Read the model definition and answer for the solid it produces. Units are mm, in the model's axes. Face numbers are marked on the shaded views. Coordinates: 2 decimals unless noted, no trailing zeros. Write each loop counter-clockwise with the first axis right and the second up, starting at its lowest first coordinate (ties: lowest second). Pieces come first, ordered by that corner, then holes.
(1) The part is cut by section D-D, the plane z = -8. Determine the outline of the cut face in (x, y), and give its area (3 significant figures).
(2) The part is cut by section C-C, the plane x = -14.25. Determine the outline of the cut face in (y, z), and give its area (3 significant figures).
(3) The part is cut by section A-A, the plane x = 0. Determine the outline of the cut face in (y, z).
(4) Given pin 1 (3 mm diameter, centred on y = 69, z = -3, fed in from -X); pin 2 (4 mm diameter, centred on y = 16, z = -0.5, fed in from -X), each flat-ended and moving along its own axis, determine where each tip first touches the part or whether it passes through.
(5) Straight lines are drawn through the part: line 1 along Z through (x, y) = (0.5, 81); line 2 along Y through (x, z) = (0, 0.65); line 3 along X through (y, z) = (60, -0.5). For each, find the intervals that lie inside material, in ascending order.
(6) The part is cut by section B-B, the plane y = -17.5. Determine the outline of the cut face in (x, z), and give its area (3 significant figures).
(7) Determine the mould class of the marked faces 1, 2, 3 and 4 for opening direction Z: pulls with the +Z half, pulls with the -Z half, needs draft (parallel to the pull), parting line crosses it, or undercut.
```python
from build123d import *

# Parameters (mm, degrees)
F0_W     = 30
F0_H     = 126.4803184569
F1_DEPTH = 3
F2_W     = 3
F2_H     = 126.4803184569
F3_DEPTH = 30
F4_START = -24
F4_DEPTH = 3


with BuildPart() as f1:
    # F0 (on Top) → F1 (new body)
    with BuildSketch(Plane.XY):
        with Locations((-3, 28.2401592284)):
            Rectangle(F0_W, F0_H)
        with BuildLine():
            ThreePointArc((-6.2781745931, -7.7781745931), (-9.1639938918, -8.3521997416), (-6.7175144213, -6.7175144213))
            ThreePointArc((-6.7175144213, -6.7175144213), (-6.3923552943, -7.2041494445), (-6.2781745931, -7.7781745931))
        make_face(mode=Mode.SUBTRACT)
        with BuildLine():
            ThreePointArc((-3.5355339059, -3.5355339059), (-1.9134171618, 4.6193976626), (5, 0))
            ThreePointArc((5, 0), (1.9134171618, -4.6193976626), (-3.5355339059, -3.5355339059))
        make_face(mode=Mode.SUBTRACT)
    extrude(amount=F1_DEPTH)

    # F2 (on face) → F3 (join)
    with BuildSketch(Plane.XY.offset(3)):
        with Locations((10.5, 28.2401592284)):
            Rectangle(F2_W, F2_H)
    extrude(amount=-F3_DEPTH)

    # F0 (on Top) → F4 (join)
    with BuildSketch(Plane.XY.offset(F4_START)):
        with Locations((-3, 28.2401592284)):
            Rectangle(F0_W, F0_H)
        with BuildLine():
            ThreePointArc((-6.2781745931, -7.7781745931), (-9.1639938918, -8.3521997416), (-6.7175144213, -6.7175144213))
            ThreePointArc((-6.7175144213, -6.7175144213), (-6.3923552943, -7.2041494445), (-6.2781745931, -7.7781745931))
        make_face(mode=Mode.SUBTRACT)
        with BuildLine():
            ThreePointArc((-3.5355339059, -3.5355339059), (-1.9134171618, 4.6193976626), (5, 0))
            ThreePointArc((5, 0), (1.9134171618, -4.6193976626), (-3.5355339059, -3.5355339059))
        make_face(mode=Mode.SUBTRACT)
        with BuildLine():
            ThreePointArc((-3.5355339059, -3.5355339059), (1.9134171618, -4.6193976626), (5, 0))
            ThreePointArc((5, 0), (-1.9134171618, 4.6193976626), (-3.5355339059, -3.5355339059))
        make_face()
        with BuildLine():
            ThreePointArc((-6.2781745931, -7.7781745931), (-6.3923552943, -7.2041494445), (-6.7175144213, -6.7175144213))
            ThreePointArc((-6.7175144213, -6.7175144213), (-9.1639938918, -8.3521997416), (-6.2781745931, -7.7781745931))
        make_face()
    extrude(amount=-F4_DEPTH)


solid = f1.part
```
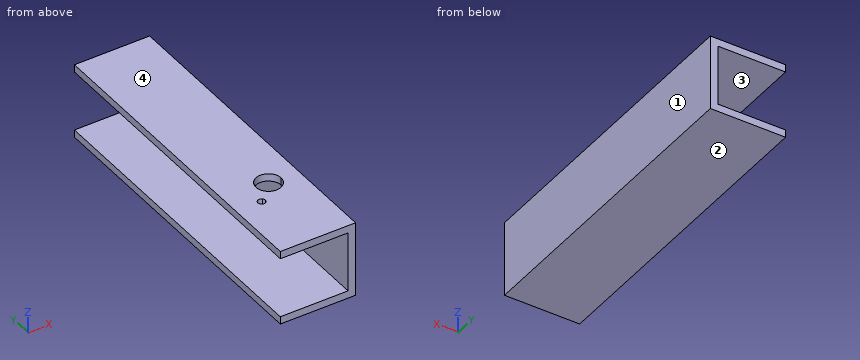
Computed:
1. outline: (9, -35) - (12, -35) - (12, 91.48) - (9, 91.48) - close
1. area: 379 mm2
2. outline: (-35, -27) - (91.48, -27) - (91.48, -24) - (-35, -24) - close; (-35, 0) - (91.48, 0) - (91.48, 3) - (-35, 3) - close
2. area: 759 mm2
3. outline: (-35, -27) - (91.48, -27) - (91.48, -24) - (-35, -24) - close; (-35, 0) - (-5, 0) - (-5, 3) - (-35, 3) - close; (5, 0) - (91.48, 0) - (91.48, 3) - (5, 3) - close
4. pin 1: stops at x = 9
4. pin 2: stops at x = -18
5. line 1: z = -27 to -24, 0 to 3
5. line 2: y = -35 to -5, 5 to 91.48
5. line 3: x = 9 to 12
6. outline: (-18, -27) - (12, -27) - (12, 3) - (-18, 3) - (-18, 0) - (9, 0) - (9, -24) - (-18, -24) - close
6. area: 252 mm2
7. face 1: needs draft
7. face 2: pulls with the -Z half
7. face 3: undercut
7. face 4: pulls with the +Z half
